from build123d import *

# Parameters (mm, degrees)
F0_R     = 4.0005
F1_DEPTH = 2.5


with BuildPart() as f1:
    # F0 (on Front) → F1 (new body, symmetric)
    with BuildSketch(Plane.XZ):
        with BuildLine():
            Line((29.9974, 9.8298), (0, 9.8298))
            Line((0, 9.8298), (-29.9974, 9.8298))
            ThreePointArc((-29.9974, 9.8298), (-39.8272, 0), (-29.9974, -9.8298))
            Line((-29.9974, -9.8298), (0, -9.8298))
            Line((0, -9.8298), (29.9974, -9.8298))
            ThreePointArc((29.9974, -9.8298), (39.8272, 0), (29.9974, 9.8298))
        make_face()
        with Locations((-29.9974, 0)):
            Circle(F0_R, mode=Mode.SUBTRACT)
        with BuildLine():
            ThreePointArc((33.9979, 0), (29.9974, -4.0005), (25.9969, 0))
            ThreePointArc((25.9969, 0), (29.9974, 4.0005), (33.9979, 0))
        make_face(mode=Mode.SUBTRACT)
    extrude(amount=F1_DEPTH, both=True)


solid = f1.part
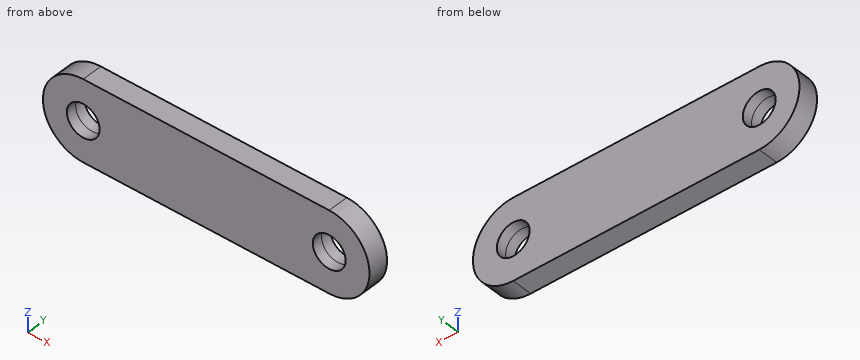
The model under review builds one solid part; all positions refer to its coordinate system, in mm. Coordinates: 2 decimals unless noted, no trailing zeros. Loops run counter-clockwise (first coordinate to the right, second up) from the corner with the lowest first, then second, coordinate; pieces in that order, holes last. Notation, with made-up numbers: (36.5, 18) -> (49.5, 18) arc R14 ccw to (49.5, 31) -> close; hole circle Ø4 at (-40, -6.75). An arc over 180 degrees is marked (long way). Use a Markdown table: item, result. Add a question column.
1. To check wall thickness, follow line 1 (X direction, y = -1.15, z = 0.75); line 2 (X direction, y = 0.15, z = 1.5); line 3 (X direction, y = 1.1, z = 5). State the ranges of each line that lie inside material, in increasing order.
2. Add section D-D on z = -5.5. Write out the cut boundary in (x, y), plus the area to 3 significant figures.
3. Add section B-B on x = -29. Write out the cut boundary in (y, z), plus the area to 3 significant figures.
4. Add section A-A on z = 0. Write out the cut boundary in (x, y), plus the area to 3 significant figures.
5. Add section C-C on y = 1. Write out the cut boundary in (x, z).
6. Clearance check with flat-ended pins moving along their axes: pin 1 Ø10.5 at (x, z) = (30, 0) entering from +Y; pin 2 Ø5 at (x, z) = (-30, 0) entering from -Y. State where each tip first meets the part, or that it passes through.
Returned:
| question | item | result |
|---|---|---|
| 1 | line 1 | x = -39.8 to -33.93, -26.07 to 26.07, 33.93 to 39.8 |
| 1 | line 2 | x = -39.71 to -33.71, -26.29 to 26.29, 33.71 to 39.71 |
| 1 | line 3 | x = -38.46 to 38.46 |
| 2 | outline | (-38.14, -2.5) -> (38.14, -2.5) -> (38.14, 2.5) -> (-38.14, 2.5) -> close |
| 2 | area | 381 mm² |
| 3 | outline | (-2.5, -9.83) -> (2.5, -9.83) -> (2.5, -3.87) -> (-2.5, -3.87) -> close; (-2.5, 3.87) -> (2.5, 3.87) -> (2.5, 9.83) -> (-2.5, 9.83) -> close |
| 3 | area | 59.6 mm² |
| 4 | outline | (-39.83, -2.5) -> (-34, -2.5) -> (-34, 2.5) -> (-39.83, 2.5) -> close; (-26, -2.5) -> (26, -2.5) -> (26, 2.5) -> (-26, 2.5) -> close; (34, -2.5) -> (39.83, -2.5) -> (39.83, 2.5) -> (34, 2.5) -> close |
| 4 | area | 318 mm² |
| 5 | outline | (-30, -9.83) -> (30, -9.83) arc R9.83 ccw to (30, 9.83) -> (-30, 9.83) arc R9.83 ccw to start; hole circle Ø8 at (-30, 0); hole circle Ø8 at (30, 0) |
| 6 | pin 1 | stops at y = 2.5 |
| 6 | pin 2 | passes through |
